from build123d import *

# Parameters (mm, degrees)
BOSS_EXTRU_1_DEPTH          = 60
ENL_V_START                 = -4
ENL_V_MAT_EXTRU_1_OUTLINE_R = 2.85
ENL_V_MAT_EXTRU_1_DEPTH     = 4
ESQUISSE3_R                 = 5.5
ENL_V_MAT_EXTRU_2_DEPTH     = 2.8
ESQUISSE4_R                 = 2.85
ENL_V_MAT_EXTRU_3_DEPTH     = 20
ESQUISSE5_R                 = 5.5
ENL_V_MAT_EXTRU_4_DEPTH     = 2.8
ESQUISSE6_W                 = 4
ESQUISSE6_H                 = 32
BOSS_EXTRU_2_DEPTH          = 31
CHANFREIN1_SIZE             = 4
ESQUISSE7_R                 = 11.75
ENL_V_MAT_EXTRU_5_DEPTH     = 4
ESQUISSE9_W                 = 4
ESQUISSE9_H                 = 28
ENL_V_MAT_EXTRU_6_DEPTH     = 20
BOSS_EXTRU_4_DEPTH          = 32
ENL_V_MAT_EXTRU_7_REACH     = 82.975
ESQUISSE11_R                = 1.9
ENL_V_START_2               = -6
ESQUISSE12_R                = 3.75
ENL_V_MAT_EXTRU_8_DEPTH     = 20
CHANFREIN2_SIZE             = 4
ESQUISSE13_W                = 14
ESQUISSE13_H                = 32
ENL_V_MAT_EXTRU_9_DEPTH     = 2
BOSS_EXTRU_5_START          = 6
BOSS_EXTRU_5_DEPTH          = 6
CHANFREIN3_SIZE             = 7
CHANFREIN4_SIZE             = 2
ESQUISSE15_W                = 11
ESQUISSE15_H                = 5
ENL_V_MAT_EXTRU_10_DEPTH    = 10


# Read off the part's stored shape, not the designer's step: Enlèv. mat.-Extru.1
# Some blends are built 0.0001 mm under size
with BuildPart() as part:
    # Esquisse1 → Boss.-Extru.1 (new body)
    with BuildSketch(Plane.XY):
        Polygon((0, 0), (0, 46), (4, 46), (4, 4), (25, 4), (25, 0), align=None)
    extrude(amount=BOSS_EXTRU_1_DEPTH)

    # Enlèv. mat.-Extru.1 outline → Enlèv. mat.-Extru.1 (cut)
    with BuildSketch(Plane(origin=(0, 4, 0), x_dir=(1, 0, 0), z_dir=(0, 1, 0)).offset(ENL_V_START)):
        with Locations((12, -9)):
            Circle(ENL_V_MAT_EXTRU_1_OUTLINE_R)
        with Locations((12, -51)):
            Circle(ENL_V_MAT_EXTRU_1_OUTLINE_R)
    extrude(amount=ENL_V_MAT_EXTRU_1_DEPTH, mode=Mode.SUBTRACT)

    # Esquisse3 → Enlèv. mat.-Extru.2 (cut)
    with BuildSketch(Plane(origin=(0, 4, 0), x_dir=(1, 0, 0), z_dir=(0, 1, 0))):
        with Locations(Location((12, -9, 0), (0, 0, 180))):
            Circle(ESQUISSE3_R)
        with Locations(Location((12, -51, 0), (0, 0, 180))):
            Circle(ESQUISSE3_R)
    extrude(amount=-ENL_V_MAT_EXTRU_2_DEPTH, mode=Mode.SUBTRACT)

    # Esquisse4 → Enlèv. mat.-Extru.3 (cut)
    with BuildSketch(Plane(origin=(4, 0, 0), x_dir=(0, 0, -1), z_dir=(1, 0, 0))):
        with Locations(Location((-51, 16, 0), (0, 0, 90))):
            Circle(ESQUISSE4_R)
        with Locations(Location((-9, 16, 0), (0, 0, 90))):
            Circle(ESQUISSE4_R)
    extrude(amount=-ENL_V_MAT_EXTRU_3_DEPTH, mode=Mode.SUBTRACT)

    # Esquisse5 → Enlèv. mat.-Extru.4 (cut)
    with BuildSketch(Plane(origin=(4, 0, 0), x_dir=(0, 0, -1), z_dir=(1, 0, 0))):
        with Locations(Location((-51, 16, 0), (0, 0, 90))):
            Circle(ESQUISSE5_R)
        with Locations(Location((-9, 16, 0), (0, 0, 90))):
            Circle(ESQUISSE5_R)
    extrude(amount=-ENL_V_MAT_EXTRU_4_DEPTH, mode=Mode.SUBTRACT)

    # Esquisse6 → Boss.-Extru.2 (add)
    with BuildSketch(Plane.XZ):
        with Locations((27, 16)):
            Rectangle(ESQUISSE6_W, ESQUISSE6_H)
    extrude(amount=-BOSS_EXTRU_2_DEPTH)

    # Chanfrein1
    chanfrein1_edges = [part.edges().sort_by_distance(p)[0] for p in [
        (25, 2, 32),
    ]]
    chamfer(chanfrein1_edges, length=CHANFREIN1_SIZE - 0.0001)  # a hair under: the kernel refuses the full size

    # Esquisse7 → Enlèv. mat.-Extru.5 (cut)
    with BuildSketch(Plane(origin=(29, 0, 0), x_dir=(0, 0, -1), z_dir=(1, 0, 0))):
        with Locations((-16, 31)):
            Circle(ESQUISSE7_R)
    extrude(amount=-ENL_V_MAT_EXTRU_5_DEPTH, mode=Mode.SUBTRACT)

    # Esquisse9 → Enlèv. mat.-Extru.6 (cut)
    with BuildSketch(Plane(origin=(0, 46, 0), x_dir=(1, 0, 0), z_dir=(0, 1, 0))):
        with Locations((2, -46)):
            Rectangle(ESQUISSE9_W, ESQUISSE9_H)
    extrude(amount=-ENL_V_MAT_EXTRU_6_DEPTH, mode=Mode.SUBTRACT)

    # Esquisse10 → Boss.-Extru.4 (add)
    with BuildSketch(Plane.XY.offset(32)):
        Polygon((0, 29), (-10, 39), (-10, 46), (0, 46), (4, 46), (4, 26), (0, 26), align=None)
    extrude(amount=-BOSS_EXTRU_4_DEPTH)

    # Enlèv. mat.-Extru.7: up to this plane
    enl_v_mat_extru_7_end = Plane(origin=(0, 29, 0), z_dir=(-0.7071067811865436, -0.7071067811865517, 0))
    # Esquisse11 → Enlèv. mat.-Extru.7 (cut, up to the surface)
    with BuildSketch(Plane(origin=(0, 46, 0), x_dir=(1, 0, 0), z_dir=(0, 1, 0)), mode=Mode.PRIVATE) as enl_v_mat_extru_7_sk1:
        with Locations(Location((-4.1, -7, 0), (0, 0, 270))):
            Circle(ESQUISSE11_R)
    enl_v_mat_extru_7_tool1 = split(extrude(enl_v_mat_extru_7_sk1.sketch, amount=-ENL_V_MAT_EXTRU_7_REACH, mode=Mode.PRIVATE), bisect_by=enl_v_mat_extru_7_end, keep=Keep.BOTH, mode=Mode.PRIVATE)
    add(enl_v_mat_extru_7_tool1.solids().sort_by_distance((-4.1, 46, 7))[0], mode=Mode.SUBTRACT)
    # Esquisse11 → Enlèv. mat.-Extru.7 (cut, up to the surface)
    with BuildSketch(Plane(origin=(0, 46, 0), x_dir=(1, 0, 0), z_dir=(0, 1, 0)), mode=Mode.PRIVATE) as enl_v_mat_extru_7_sk2:
        with Locations(Location((-4.1, -25, 0), (0, 0, 270))):
            Circle(ESQUISSE11_R)
    enl_v_mat_extru_7_tool2 = split(extrude(enl_v_mat_extru_7_sk2.sketch, amount=-ENL_V_MAT_EXTRU_7_REACH, mode=Mode.PRIVATE), bisect_by=enl_v_mat_extru_7_end, keep=Keep.BOTH, mode=Mode.PRIVATE)
    add(enl_v_mat_extru_7_tool2.solids().sort_by_distance((-4.1, 46, 25))[0], mode=Mode.SUBTRACT)

    # Esquisse12 → Enlèv. mat.-Extru.8 (cut)
    with BuildSketch(Plane(origin=(0, 46, 0), x_dir=(1, 0, 0), z_dir=(0, 1, 0)).offset(ENL_V_START_2)):
        with Locations(Location((-4.1, -7, 0), (0, 0, 270))):
            Circle(ESQUISSE12_R)
        with Locations(Location((-4.1, -25, 0), (0, 0, 270))):
            Circle(ESQUISSE12_R)
    extrude(amount=-ENL_V_MAT_EXTRU_8_DEPTH, mode=Mode.SUBTRACT)

    # Chanfrein2
    chanfrein2_edges = [part.edges().sort_by_distance(p)[0] for p in [
        (2, 26, 60),
        (25, 2, 60),
    ]]
    chamfer(chanfrein2_edges, length=CHANFREIN2_SIZE)

    # Esquisse13 → Enlèv. mat.-Extru.9 (cut)
    with BuildSketch(Plane(origin=(0, 46, 0), x_dir=(1, 0, 0), z_dir=(0, 1, 0))):
        with Locations((-3, -16)):
            Rectangle(ESQUISSE13_W, ESQUISSE13_H)
    extrude(amount=-ENL_V_MAT_EXTRU_9_DEPTH, mode=Mode.SUBTRACT)

    # Esquisse14 → Boss.-Extru.5 (add)
    with BuildSketch(Plane(origin=(29, 0, 0), x_dir=(0, 0, -1), z_dir=(1, 0, 0)).offset(BOSS_EXTRU_5_START)):
        with BuildLine():
            Line((-32, 31), (-27.75, 31))
            ThreePointArc((-27.75, 31), (-16, 19.25), (-4.25, 31))
            Line((-4.25, 31), (0, 31))
            ThreePointArc((0, 31), (-16, 15), (-32, 31))
        make_face()
    extrude(amount=-BOSS_EXTRU_5_DEPTH)

    # Chanfrein3
    # the kernel refuses this chamfer: 7 mm, written as the material it adds along each edge
    with BuildSketch(Plane(origin=(29, 31, 16), x_dir=(0, 0, -1), z_dir=(0, 1, 0))) as chanfrein3_piece_1_section:
        Polygon((16 + CHANFREIN3_SIZE, 0), (16, -CHANFREIN3_SIZE), (16, 0), align=None)
    chanfrein3_piece_1 = revolve(axis=Axis((29, 31, 16), (-1, 0, 0)), revolution_arc=180, mode=Mode.PRIVATE)
    chanfrein3_piece_1 = split(chanfrein3_piece_1, bisect_by=Plane(origin=(32, 14.901456645, 32), z_dir=(0, 0, -1)), keep=Keep.TOP, mode=Mode.PRIVATE)
    chanfrein3_piece_1 = split(chanfrein3_piece_1, bisect_by=Plane(origin=(32, 14.901456645, 0), z_dir=(0, 0, 1)), keep=Keep.TOP, mode=Mode.PRIVATE)
    chanfrein3_piece_1 = split(chanfrein3_piece_1, bisect_by=Plane(origin=(35, 14.901456645, 16), z_dir=(-1, 0, 0)), keep=Keep.TOP, mode=Mode.PRIVATE)
    add(chanfrein3_piece_1)

    # Chanfrein4
    chanfrein4_edges = [part.edges().sort_by_distance(p)[0] for p in [
        (35, 19.25, 16),
    ]]
    chamfer(chanfrein4_edges, length=CHANFREIN4_SIZE)

    # Esquisse15 → Enlèv. mat.-Extru.10 (cut)
    with BuildSketch(Plane(origin=(0, 4, 0), x_dir=(1, 0, 0), z_dir=(0, 1, 0))):
        with Locations((14.5, -25)):
            Rectangle(ESQUISSE15_W, ESQUISSE15_H)
        with Locations((14.5, -35)):
            Rectangle(ESQUISSE15_W, ESQUISSE15_H)
    extrude(amount=-ENL_V_MAT_EXTRU_10_DEPTH, mode=Mode.SUBTRACT)


solid = part.part
Geometry check sheet. Reference: the model listing, model coordinates, mm. A direction names the side the tool comes from. Round coordinates to 2 decimals unless told otherwise and drop trailing zeros. Loops run counter-clockwise (first coordinate to the right, second up) from the corner with the lowest first, then second, coordinate; pieces in that order, holes last. Notation, with made-up numbers: (-32, 10.25) - (-5, 10.25) arc R25 ccw to (-5, 49.25) - close; hole circle Ø2 at (-4, 22.5). An arc over 180 degrees is marked (long way). One line per question, with ' | ' between items. Start each with the question number.
1. Cross-section at A-A on z = 51. Record the cut outline in (x, y), then the cut area to 3 significant figures.
2. Cross-section at B-B on x = 12. Record the cut outline in (y, z), then the cut area to 3 significant figures.
3. Cross-section at D-D on x = -4.1. Record the cut outline in (y, z), then the cut area to 3 significant figures.
4. Scan lines: line 1 (Z direction, x = -4, y = 41); line 2 (Z direction, x = 12, y = 3.1); line 3 (Z direction, x = -4, y = 35). Record each from-to range of solid material in increasing order. Write a range as [from, to].
5. Depth check by flat-ended pin: pin 1 (4 mm diameter, centred on y = 7.5, z = 29, fed in from -X); pin 2 (6 mm diameter, centred on x = -4.5, z = 38, fed in from -Y); pin 3 (4 mm diameter, centred on x = -1, y = 35.5, fed in from +Z); pin 4 (10 mm diameter, centred on x = 12, z = 9, fed in from +Y). Enter the tip coordinate at first touch or a pass-through.
6. Tool access check on faces 1 (the face through (9, 2, 35)), 2 (the face through (-3, 40, 5)), 3 (the face through (25, 14, 16)), 4 (the face through (29, 19, 32)), 5 (the face through (9.5, 2.6, 4.1)). Record the directions out of +Z, -Z, +X, -X, +Y, -Y that give a thin tool (end or side, any length) a straight path to the whole face; none if there is none.
7. Cross-section at C-C on y = 5. Record the cut outline in (x, z).
8. Draft check along Y on faces 6 (the face through (25, 2, 46)), 7 (the face through (0.608, 13.899, 10.926)), 8 (the face through (-5, 34, 16)). Enter one of: released by +Y, released by -Y, zero draft, split by the parting line, or undercut.
Taken from the geometry:
1) outline: (0, 0) - (9.15, 0) - (9.15, 1.2) - (6.5, 1.2) - (6.5, 4) - (4, 4) - (4, 10.5) - (1.2, 10.5) - (1.2, 13.15) - (0, 13.15) - close; (0, 18.85) - (1.2, 18.85) - (1.2, 21.5) - (4, 21.5) - (4, 26) - (0, 26) - close; (14.85, 0) - (25, 0) - (25, 4) - (17.5, 4) - (17.5, 1.2) - (14.85, 1.2) - close | area: 113 mm²
2) outline: (0, 0) - (4, 0) - (4, 3.5) - (1.2, 3.5) - (1.2, 6.15) - (0, 6.15) - close; (0, 11.85) - (1.2, 11.85) - (1.2, 14.5) - (4, 14.5) - (4, 22.5) - (0, 22.5) - close; (0, 27.5) - (4, 27.5) - (4, 32.5) - (0, 32.5) - close; (0, 37.5) - (4, 37.5) - (4, 45.5) - (1.2, 45.5) - (1.2, 48.15) - (0, 48.15) - close; (0, 53.85) - (1.2, 53.85) - (1.2, 56.5) - (4, 56.5) - (4, 60) - (0, 60) - close | area: 125 mm²
3) outline: (33.1, 0) - (44, 0) - (44, 5.1) - (40, 5.1) - (40, 3.25) - (33.1, 3.25) - close; (33.1, 10.75) - (40, 10.75) - (40, 8.9) - (44, 8.9) - (44, 23.1) - (40, 23.1) - (40, 21.25) - (33.1, 21.25) - close; (33.1, 28.75) - (40, 28.75) - (40, 26.9) - (44, 26.9) - (44, 32) - (33.1, 32) - close | area: 215 mm²
4) line 1: [0, 5.1], [8.9, 23.1], [26.9, 32] | line 2: [0, 3.5], [14.5, 22.5], [27.5, 32.5], [37.5, 45.5], [56.5, 60] | line 3: [0, 3.25], [10.75, 21.25], [28.75, 32]
5) pin 1: x = 0 | pin 2: through | pin 3: z = 32 | pin 4: y = 1.2
6) face 1: +Y, -Y | face 2: -Y | face 3: +Z, -Z, +Y | face 4: +Z, +X, +Y | face 5: +Y
7) outline: (0, 0) - (4, 0) - (4, 60) - (0, 60) - close; (25, 0) - (29, 0) - (29, 32) - (25, 32) - close
8) face 6: zero draft | face 7: undercut | face 8: released by -Y
